Check sheet for the modelled part. Datum: model origin and axes. Units: mm. A direction names the side the tool comes from. Round coordinates to 2 decimals unless told otherwise and drop trailing zeros. Order: outer loops, then holes, each group sorted by start corner. A loop starts at its lowest first (then second) coordinate and runs counter-clockwise, first axis right, second up.
Q1. Mould release check, pull along X, two halves, no side actions. Record for faces 5 (the flat face through (0, 0, 0)), 6 (the flat face through (0, 27, 27.335)), 7 (the cylindrical face through (-16.5, 24.4, -20.3)), 8 (the flat face through (19, 23, 0)): +X half, -X half, draft (parallel to the pull), parting line (faces both ways), or undercut.
Q2. Cross-section at C-C on x = -20. Record the cut outline in (y, z), then the cut area to 3 significant figures.
Q3. Set-up check for faces 1 (the cylindrical face through (19.394, -1.479, -12.365)), 2 (the cylindrical face through (16.5, 24.4, 20.3)), 3 (the cylindrical face through (-21.46, 42.44, 0.54)), 4 (the flat face through (24, 40, 0)): record each of +Z, -Z, +X, -X, +Y, -Y from which the full face is reachable in a straight line by a thin tool's end or side.
Q4. Cross-section at D-D on x = -5. Record the cut outline in (y, z), then the cut area to 3 significant figures.
Q5. Cross-section at B-B on y = 4.5. Record the cut outline in (x, z), then the cut area to 3 significant figures.
Q6. Depth check by flat-ended pin: P1, Ø14, axis at y = 26.5, z = -1.5, coming from the -X side; P2, Ø2.5, axis at y = 41, z = -1, coming from the +X side; P3, Ø4, axis at x = -20.5, z = -9, coming from the -Y side; P4, Ø3, axis at x = -14.5, y = 13.5, coming from the -Z side. Enter the tip coordinate at first touch or a pass-through.
Q7. Cross-section at A-A on z = 0. Record the cut outline in (x, y), then the cut area to 3 significant figures.
Q8. Scan lines: probe 1 along X at (y, z) = (-1.6, 0); probe 2 along X at (y, z) = (7.5, 12); probe 3 along Y at (x, z) = (3, 9). Record each from-to range of solid material in increasing order.
from build123d import *

# Parameters (mm, degrees)
SKETCH1_R           = 27.5
BOSS_EXTRUDE1_DEPTH = 2
SKETCH2_R           = 25
SKETCH2_R_2         = 23
BOSS_EXTRUDE2_DEPTH = 3
BOSS_EXTRUDE3_DEPTH = 50.8
CHAMFER1_SIZE       = 21.979819356
CHAMFER1_SIZE_2     = 8
SKETCH4_R           = 2.5
BOSS_EXTRUDE4_DEPTH = 5


with BuildPart() as part:
    # Sketch1 → Boss-Extrude1 (new body)
    with BuildSketch(Plane(origin=(0, 0, 0), x_dir=(1, 0, 0), z_dir=(0, 1, 0))):
        with Locations(Location((0, 0, 0), (0, 0, 270))):
            Circle(SKETCH1_R)
    extrude(amount=BOSS_EXTRUDE1_DEPTH)

    # Sketch2 → Boss-Extrude2 (add)
    with BuildSketch(Plane.XZ):
        with Locations(Location((0, 0, 0), (0, 0, 90))):
            Circle(SKETCH2_R)
        with Locations(Location((0, 0, 0), (0, 0, 270))):
            Circle(SKETCH2_R_2, mode=Mode.SUBTRACT)
    extrude(amount=BOSS_EXTRUDE2_DEPTH)

    # Sketch3 → Boss-Extrude3 (add)
    with BuildSketch(Plane(origin=(0, 2, 0), x_dir=(1, 0, 0), z_dir=(0, 1, 0))):
        with BuildLine():
            ThreePointArc((-11.903598775, 24.790206457), (-16.564617944, 20.201602313), (-19, 14.131239727))
            Line((-19, 14.131239727), (-19, -14.131239727))
            ThreePointArc((-19, -14.131239727), (-16.564617944, -20.201602313), (-11.903598775, -24.790206457))
            ThreePointArc((-11.903598775, -24.790206457), (-7.564953068, -26.43901445), (-3.010813341, -27.334684981))
            Line((-3.010813341, -27.334684981), (3.010813341, -27.334684981))
            ThreePointArc((3.010813341, -27.334684981), (7.564953068, -26.43901445), (11.903598775, -24.790206457))
            ThreePointArc((11.903598775, -24.790206457), (16.564617944, -20.201602313), (19, -14.131239727))
            Line((19, -14.131239727), (19, 14.131239727))
            ThreePointArc((19, 14.131239727), (16.564617944, 20.201602313), (11.903598775, 24.790206457))
            ThreePointArc((11.903598775, 24.790206457), (7.564953068, 26.43901445), (3.010813341, 27.334684981))
            Line((3.010813341, 27.334684981), (-3.010813341, 27.334684981))
            ThreePointArc((-3.010813341, 27.334684981), (-7.564953068, 26.43901445), (-11.903598775, 24.790206457))
        make_face()
    extrude(amount=BOSS_EXTRUDE3_DEPTH)

    # Chamfer1
    # the kernel refuses this chamfer: 21.979819356, 8 mm, written as the material it takes off along each edge
    with BuildSketch(Plane(origin=(19, 52.8, 71.151171322), x_dir=(-0.9999130865277316, 0.013184058198645697, 0), z_dir=(0, 0, -1)), Plane(origin=(-19, 52.8, -71.151171322), x_dir=(0.9999130865277316, 0.013184058198645697, 0), z_dir=(0, 0, 1))) as chamfer1_piece_1:
        Polygon((CHAMFER1_SIZE * 0.999913086511, -CHAMFER1_SIZE * 0.0131840581984), (-CHAMFER1_SIZE_2 * 0.0131840581986, -CHAMFER1_SIZE_2 * 0.999913086528), (0, 0), align=None)
    extrude(amount=142.302342643, mode=Mode.SUBTRACT)

    # Sketch4 → Boss-Extrude4 (add)
    with BuildSketch(Plane.ZY.offset(19)):
        with Locations(Location((0, 40, 0), (0, 0, 180))):
            Circle(SKETCH4_R)
    boss_extrude4 = extrude(amount=BOSS_EXTRUDE4_DEPTH)

    # Mirror1: Boss-Extrude4 across plane
    add(boss_extrude4.mirror(Plane(origin=(0, 0, 0), x_dir=(0, 0, 1), z_dir=(1, 0, 0))))


solid = part.part
Results found:
1. face 5: undercut
1. face 6: draft
1. face 7: -X half
1. face 8: +X half
2. outline: (-3, -15) - (0, -15) - (0, -18.87) - (2, -18.87) - (2, 18.87) - (0, 18.87) - (0, 15) - (-3, 15) - (-3, 11.36) - (0, 11.36) - (0, -11.36) - (-3, -11.36) - close; circle Ø5 at (40, 0)
2. area: 117 mm2
3. face 1: -Y
3. face 2: +Z, +X, +Y
3. face 3: -X
3. face 4: +Z, -Z, +X, +Y
4. outline: (-3, -24.49) - (0, -24.49) - (0, -27.04) - (49.9, -27.04) - (49.9, 27.04) - (0, 27.04) - (0, 24.49) - (-3, 24.49) - (-3, 22.45) - (0, 22.45) - (0, -22.45) - (-3, -22.45) - close
4. area: 2,710 mm2
5. outline: (-19, -14.13) arc R16 ccw to (-11.9, -24.79) arc R27.5 ccw to (-3.01, -27.33) - (3.01, -27.33) arc R27.5 ccw to (11.9, -24.79) arc R16 ccw to (19, -14.13) - (19, 14.13) arc R16 ccw to (11.9, 24.79) arc R27.5 ccw to (3.01, 27.33) - (-3.01, 27.33) arc R27.5 ccw to (-11.9, 24.79) arc R16 ccw to (-19, 14.13) - close
5. area: 1,860 mm2
6. P1: stops at x = -19
6. P2: stops at x = 24
6. P3: stops at y = -3
6. P4: stops at z = -24.02
7. outline: (-27.5, 0) - (-25, 0) - (-25, -3) - (-23, -3) - (-23, 0) - (23, 0) - (23, -3) - (25, -3) - (25, 0) - (27.5, 0) - (27.5, 2) - (19, 2) - (19, 37.5) - (24, 37.5) - (24, 42.5) - (19, 42.5) - (19, 44.8) - (0, 51.72) - (-19, 44.8) - (-19, 42.5) - (-24, 42.5) - (-24, 37.5) - (-19, 37.5) - (-19, 2) - (-27.5, 2) - close
7. area: 1,930 mm2
8. probe 1: x = -25 to -23, 23 to 25
8. probe 2: x = -19 to 19
8. probe 3: y = 0 to 50.62
